from build123d import *

# Parameters (mm, degrees)
SFAZOWANIE1_SIZE = 1
SFAZOWANIE2_SIZE = 1


with BuildPart() as part:
    # Szkic1 → Obrót1 (revolve)
    with BuildSketch(Plane(origin=(0, 0, 0), x_dir=(0, 0, -1), z_dir=(1, 0, 0)), mode=Mode.PRIVATE) as obr_t1_sk:
        Polygon((0, 0), (300, 0), (300, 6), (284, 6), (284, 8), (52, 8), (52, 6), (22, 6), (22, 5), (9, 5), (9, 4), (0, 4), align=None)
    revolve(obr_t1_sk.sketch.rotate(Axis((0, 0, 0), (0, 0, -1)), 90), axis=Axis((0, 0, 0), (0, 0, -1)))

    # Sfazowanie1
    sfazowanie1_edges = [part.edges().sort_by_distance(p)[0] for p in [
        (-6, 0, -22),
        (-4, 0, 0),
        (-5, 0, -9),
    ]]
    chamfer(sfazowanie1_edges, length=SFAZOWANIE1_SIZE - 0.0001)  # a hair under: the kernel refuses the full size

    # Sfazowanie2
    sfazowanie2_edges = [part.edges().sort_by_distance(p)[0] for p in [
        (-6, 0, -300),
    ]]
    chamfer(sfazowanie2_edges, length=SFAZOWANIE2_SIZE)


solid = part.part
The listing builds one solid part. Answer for the finished solid, in the listing's coordinates (mm). A direction names the side the tool comes from. Round coordinates to 2 decimals unless told otherwise and drop trailing zeros. Loops run counter-clockwise (first coordinate to the right, second up) from the corner with the lowest first, then second, coordinate; pieces in that order, holes last. Notation, with made-up numbers: M 8.5,-2.75 L 18.5,-2.75 A27 ccw 18.5,31.25 Z; hole C -12.75,-25.5 d3. An arc over 180 degrees is marked long. Write each question's results on one line, items separated by ' | '. Start each with the question number.
1) Find section C-C on z = -108. Write down the section's boundary in (x, y), plus the area to 3 significant figures.
2) Each of these flat-tipped pins is pushed along its axis until it touches: pin 1 (8 mm diameter, centred on x = -6, z = -40.5, fed in from -Y); pin 2 (5 mm diameter, centred on x = -2, y = 0.5, fed in from +Z); pin 3 (2 mm diameter, centred on y = 5, z = -162.5, fed in from -X); pin 4 (1 mm diameter, centred on y = -5, z = -100.5, fed in from -X). Where does it stop, or does it pass through?
3) Straight lines are drawn through the part: probe 1 along Y at (x, z) = (-0.75, -140.5); probe 2 along X at (y, z) = (0.5, -85.5); probe 3 along Z at (x, y) = (1, -7.5). For each, find the intervals that lie inside material, in ascending order.
4) Which of the six approach directions +Z, -Z, +X, -X, +Y, -Y give full straight-line access (tool end or side, diameter ignored) to faces 1 (the flat face through (-2, -6, -52)), 2 (the cylindrical face through (5.723, -1.802, -291.395)), 3 (the flat face through (0, 0, -300))?
5) Find section D-D on z = -28. Write down the section's boundary in (x, y), plus the area to 3 significant figures.
Final values:
1) outline: C 0,0 d16 | area: 201 mm²
2) pin 1: y = -5.66 | pin 2: z = 0 | pin 3: x = -6.93 | pin 4: x = -6.61
3) probe 1: -7.96 to 7.96 | probe 2: -7.98 to 7.98 | probe 3: -284 to -52
4) face 1: +Z | face 2: -Z | face 3: -Z, +X, -X, +Y, -Y
5) outline: C 0,0 d12 | area: 113 mm²
